For this review, use the dimensioned drawing (mm, ordinates from the lowest corner) and the shaded views. Round coordinates to 2 decimals unless told otherwise and drop trailing zeros. Write each loop counter-clockwise with the first axis right and the second up, starting at its lowest first coordinate (ties: lowest second). Pieces come first, ordered by that corner, then holes. Notation, with made-up numbers: M 87.5,31.25 L 138.5,31.25 A29 cw 138.5,51.25 Z; hole C 85.25,-27.75 d2. An arc over 180 degrees is marked long. One line per question, with ' | ' between items.
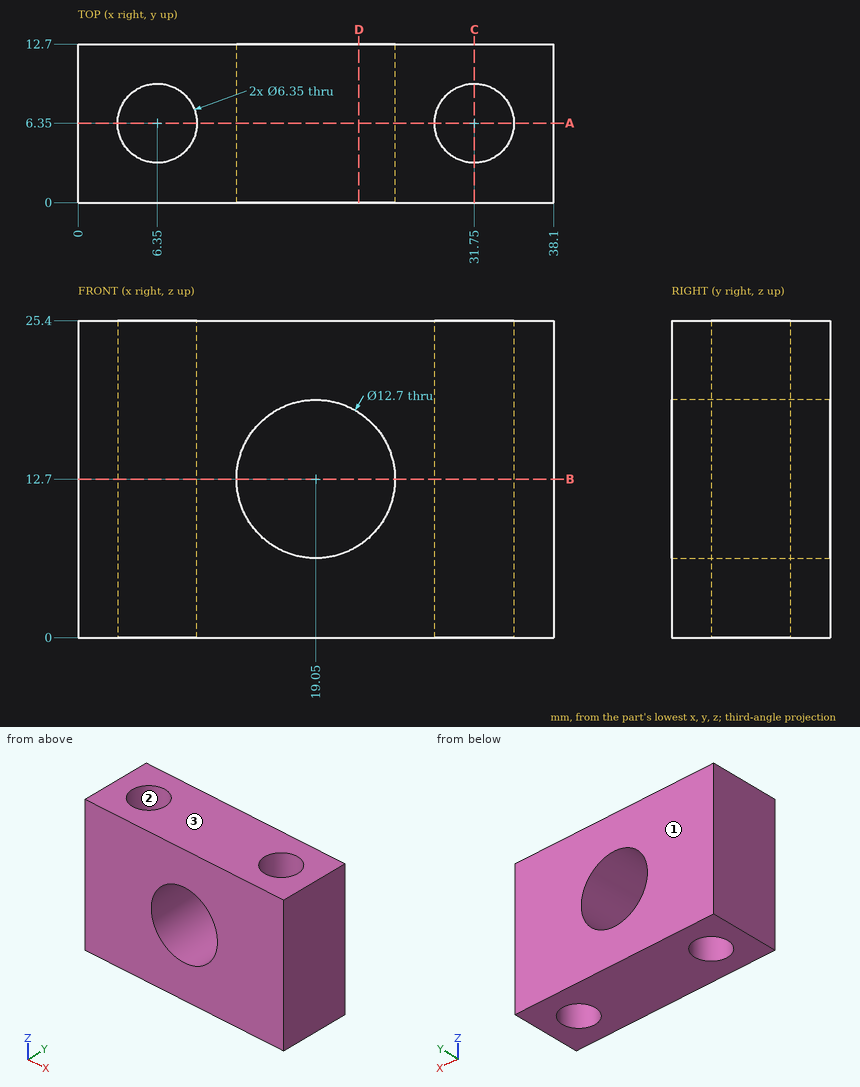
Item 1: Take a section at D-D (x = 22.5). Write out the cut boundary in (y, z), then the cut area to 3 significant figures.
Results:
outline: M 0,0 L 12.7,0 L 12.7,7.37 L 0,7.37 Z; M 0,18.03 L 12.7,18.03 L 12.7,25.4 L 0,25.4 Z | area: 187 mm2
Item 2: To check wall thickness, follow line 1 along X through (y, z) = (7.5, 8.75); line 2 along X through (y, z) = (6, 8.5); line 3 along Y through (x, z) = (31.75, 12) (3 decimals). State the ranges of each line that lie inside material, in increasing order. Write a range as from..to.
Results:
line 1: 0..3.39, 9.31..14.08, 24.02..28.79, 34.71..38.1 | line 2: 0..3.19, 9.51..14.29, 23.81..28.59, 34.91..38.1 | line 3: 0..3.175, 9.525..12.7
Item 3: Take a section at B-B (z = 12.7). Write out the cut boundary in (x, y) (3 decimals), then the cut area to 3 significant figures.
Results:
outline: M 0,0 L 12.7,0 L 12.7,12.7 L 0,12.7 Z; M 25.4,0 L 38.1,0 L 38.1,12.7 L 25.4,12.7 Z; hole C 6.35,6.35 d6.35; hole C 31.75,6.35 d6.35 | area: 259 mm2
Item 4: Mouldability with a two-part tool opening along Y and no side actions: class the marked faces 1, 2 and 3 as +Y half, -Y half, draft (parallel to the pull), parting line (faces both ways), or undercut.
Results:
face 1: +Y half | face 2: undercut | face 3: draft
Item 5: Take a section at C-C (x = 31.75). Write out the cut boundary in (y, z) (3 decimals), then the cut area to 3 significant figures.
Results:
outline: M 0,0 L 3.175,0 L 3.175,25.4 L 0,25.4 Z; M 9.525,0 L 12.7,0 L 12.7,25.4 L 9.525,25.4 Z | area: 161 mm2
Item 6: Take a section at A-A (y = 6.35). Write out the cut boundary in (x, z) (3 decimals), then the cut area to 3 significant figures.
Results:
outline: M 0,0 L 3.175,0 L 3.175,25.4 L 0,25.4 Z; M 9.525,0 L 28.575,0 L 28.575,25.4 L 9.525,25.4 Z; M 34.925,0 L 38.1,0 L 38.1,25.4 L 34.925,25.4 Z; hole C 19.05,12.7 d12.7 | area: 518 mm2
